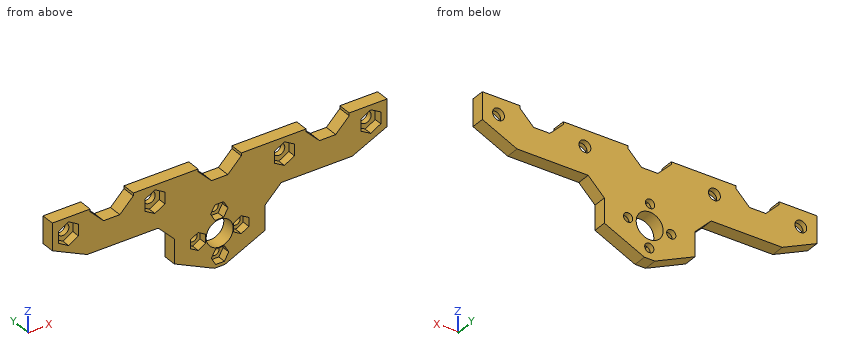
from build123d import *
from OCP.BRepFilletAPI import BRepFilletAPI_MakeChamfer

# Parameters (mm, degrees)
SKETCH1_W           = 124
SKETCH1_H           = 42
BOSS_EXTRUDE1_DEPTH = 5
SKETCH2_R           = 5
CUT_EXTRUDE1_DEPTH  = 5
SKETCH3_W           = 124
SKETCH3_H           = 42
SKETCH3_R           = 2.2
SKETCH3_R_2         = 1.7
SKETCH3_R_3         = 5
BOSS_EXTRUDE2_DEPTH = 2
CHAMFER1_SIZE       = 28
CHAMFER1_SIZE2      = 60.046193774
CUT_EXTRUDE2_DEPTH  = 10
LPATTERN1_COUNT     = 3
LPATTERN1_PITCH     = 40
SKETCH5_W           = 124
SKETCH5_H           = 4
CUT_EXTRUDE3_DEPTH  = 10
CUT_EXTRUDE4_DEPTH  = 10
CHAMFER2_SIZE       = 6


with BuildPart() as part:
    # Sketch1 → Boss-Extrude1 (new body)
    with BuildSketch(Plane.XZ.offset(-139.173467121)):
        with Locations((90.436218841, 110.61857787)):
            Rectangle(SKETCH1_W, SKETCH1_H)
        Polygon((87.341918286, 93.619783108), (88.95849904, 90.819783108), (92.191660547, 90.819783108), (93.808241301, 93.619783108), (92.191660547, 96.419783108), (88.95849904, 96.419783108), align=None, mode=Mode.SUBTRACT)
        Polygon((98.435013602, 98.524277315), (101.235013602, 100.140858069), (101.235013602, 103.374019576), (98.435013602, 104.99060033), (95.635013602, 103.374019576), (95.635013602, 100.140858069), align=None, mode=Mode.SUBTRACT)
        Polygon((82.437424079, 104.712878424), (79.637424079, 103.09629767), (79.637424079, 99.863136163), (82.437424079, 98.246555409), (85.237424079, 99.863136163), (85.237424079, 103.09629767), align=None, mode=Mode.SUBTRACT)
        Polygon((93.530519395, 109.617372631), (91.913938641, 112.417372631), (88.680777134, 112.417372631), (87.06419638, 109.617372631), (88.680777134, 106.817372631), (91.913938641, 106.817372631), align=None, mode=Mode.SUBTRACT)
        Polygon((34.436218841, 125.890969862), (30.736218841, 123.754773866), (30.736218841, 119.482381874), (34.436218841, 117.346185878), (38.136218841, 119.482381874), (38.136218841, 123.754773866), align=None, mode=Mode.SUBTRACT)
        Polygon((62.736218841, 123.754773866), (62.736218841, 119.482381874), (66.436218841, 117.346185878), (70.136218841, 119.482381874), (70.136218841, 123.754773866), (66.436218841, 125.890969862), align=None, mode=Mode.SUBTRACT)
        Polygon((118.136218841, 123.754773866), (114.436218841, 125.890969862), (110.736218841, 123.754773866), (110.736218841, 119.482381874), (114.436218841, 117.346185878), (118.136218841, 119.482381874), align=None, mode=Mode.SUBTRACT)
        Polygon((142.736218841, 119.482381874), (146.436218841, 117.346185878), (150.136218841, 119.482381874), (150.136218841, 123.754773866), (146.436218841, 125.890969862), (142.736218841, 123.754773866), align=None, mode=Mode.SUBTRACT)
    extrude(amount=BOSS_EXTRUDE1_DEPTH)

    # Sketch2 → Cut-Extrude1 (cut)
    with BuildSketch(Plane(origin=(0, 139.173467121, 0), x_dir=(1, 0, 0), z_dir=(0, 1, 0))):
        with Locations(Location((90.436218841, -101.61857787, 0), (0, 0, 270))):
            Circle(SKETCH2_R)
    extrude(amount=-CUT_EXTRUDE1_DEPTH, mode=Mode.SUBTRACT)

    # Sketch3 → Boss-Extrude2 (add)
    with BuildSketch(Plane(origin=(0, 139.173467121, 0), x_dir=(1, 0, 0), z_dir=(0, 1, 0))):
        with Locations((90.436218841, -110.61857787)):
            Rectangle(SKETCH3_W, SKETCH3_H)
        with Locations(Location((34.436218841, -121.61857787, 0), (0, 0, 270))):
            Circle(SKETCH3_R, mode=Mode.SUBTRACT)
        with Locations(Location((66.436218841, -121.61857787, 0), (0, 0, 270))):
            Circle(SKETCH3_R, mode=Mode.SUBTRACT)
        with Locations(Location((114.436218841, -121.61857787, 0), (0, 0, 270))):
            Circle(SKETCH3_R, mode=Mode.SUBTRACT)
        with Locations(Location((146.436218841, -121.61857787, 0), (0, 0, 270))):
            Circle(SKETCH3_R, mode=Mode.SUBTRACT)
        with Locations(Location((90.575079793, -93.619783108, 0), (0, 0, 270))):
            Circle(SKETCH3_R_2, mode=Mode.SUBTRACT)
        with Locations(Location((82.437424079, -101.479716917, 0), (0, 0, 270))):
            Circle(SKETCH3_R_2, mode=Mode.SUBTRACT)
        with Locations(Location((90.297357888, -109.617372631, 0), (0, 0, 270))):
            Circle(SKETCH3_R_2, mode=Mode.SUBTRACT)
        with Locations(Location((98.435013602, -101.757438823, 0), (0, 0, 270))):
            Circle(SKETCH3_R_2, mode=Mode.SUBTRACT)
        with Locations(Location((90.436218841, -101.61857787, 0), (0, 0, 270))):
            Circle(SKETCH3_R_3, mode=Mode.SUBTRACT)
    extrude(amount=-BOSS_EXTRUDE2_DEPTH)

    # Chamfer1: one chamfer whose edges measure the first distance from different faces: ONE call of the kernel's chamfer builder (chamfer() names one face for all edges)
    chamfer1_edges_1 = [part.edges().sort_by_distance(p)[0] for p in [
        (152.436218841, 136.673467121, 89.61857787),
    ]]
    chamfer1_side_1 = [part.faces().sort_by_distance(p)[0] for p in [
        (152.436218841, 136.673467121, 110.61857787),
    ]]
    chamfer1_edges_2 = [part.edges().sort_by_distance(p)[0] for p in [
        (28.436218841, 136.673467121, 89.61857787),
    ]]
    chamfer1_side_2 = [part.faces().sort_by_distance(p)[0] for p in [
        (28.436218841, 136.673467121, 110.61857787),
    ]]
    chamfer1 = BRepFilletAPI_MakeChamfer(part.part.solid().wrapped)
    for e in chamfer1_edges_1:
        chamfer1.Add(CHAMFER1_SIZE, CHAMFER1_SIZE2, e.wrapped, chamfer1_side_1[0].wrapped)  # the first distance lies on this face
    for e in chamfer1_edges_2:
        chamfer1.Add(CHAMFER1_SIZE, CHAMFER1_SIZE2, e.wrapped, chamfer1_side_2[0].wrapped)  # the first distance lies on this face
    add(Compound.cast(chamfer1.Shape()), mode=Mode.REPLACE)

    # Sketch4 → Cut-Extrude2 (cut)
    with BuildSketch(Plane.XZ.offset(-134.173467121)):
        Polygon((42.436218841, 131.61857787), (58.436218841, 131.61857787), (58.436218841, 126.61857787), (53.436218841, 121.61857787), (47.436218841, 121.61857787), (42.436218841, 126.61857787), align=None)
    cut_extrude2 = extrude(amount=-CUT_EXTRUDE2_DEPTH, mode=Mode.SUBTRACT)

    # LPattern1: Cut-Extrude2 ×3
    with Locations(*[(i * LPATTERN1_PITCH, 0, 0) for i in range(1, LPATTERN1_COUNT)]):
        add(cut_extrude2, mode=Mode.SUBTRACT)

    # Sketch5 → Cut-Extrude3 (cut)
    with BuildSketch(Plane.XZ.offset(-134.173467121)):
        with Locations((90.436218841, 129.61857787)):
            Rectangle(SKETCH5_W, SKETCH5_H)
    extrude(amount=-CUT_EXTRUDE3_DEPTH, mode=Mode.SUBTRACT)

    # Sketch6 → Cut-Extrude4 (cut)
    with BuildSketch(Plane.XZ.offset(-134.173467121)):
        Polygon((41.303260364, 111.61857787), (73.637424079, 111.61857787), (73.637424079, 96.540909709), align=None)
        Polygon((107.235013602, 111.61857787), (107.235013602, 96.540909709), (139.569177317, 111.61857787), align=None)
    extrude(amount=-CUT_EXTRUDE4_DEPTH, mode=Mode.SUBTRACT)

    # Chamfer2
    chamfer2_edges = [part.edges().sort_by_distance(p)[0] for p in [
        (73.637424079, 136.673467121, 111.61857787),
        (107.235013602, 136.673467121, 111.61857787),
    ]]
    chamfer(chamfer2_edges, length=CHAMFER2_SIZE)


solid = part.part
The listing builds one solid part. Answer for the finished solid, in the listing's coordinates (mm). Coordinates: 2 decimals unless noted, no trailing zeros. Order: outer loops, then holes, each group sorted by start corner. A loop starts at its lowest first (then second) coordinate and runs counter-clockwise, first axis right, second up.
Q1. A cutting plane is placed at B-B, the plane y = 138.3. State how many separate pieces and enclosed holes the cut face has, and give its area (3 significant figures).
Q2. Given P1, Ø2.5, axis at x = 130.5, y = 137, coming from the +Z side; P2, Ø1.5, axis at x = 132, y = 137.5, coming from the -Z side; P3, Ø1.7, axis at x = 99, z = 102.5, coming from the -Y side, each flat-ended and moving along its own axis, determine where each tip first touches the part or whether it passes through.
Q3. A cutting plane is placed at C-C, the plane x = 60. Write down the section's boundary in (y, z), and give its area (3 significant figures).
Q4. A cutting plane is placed at A-A, the plane z = 102. Write down the section's boundary in (x, y).
Q5. A cutting plane is placed at D-D, the plane z = 113.5. Write down the section's boundary in (x, y), and give its area (3 significant figures).
Q6. Consider line 1 (X direction, y = 138, z = 121.5); line 2 (X direction, y = 135.75, z = 121); line 3 (X direction, y = 136.95, z = 100.5). Determine where each line is inside the solid, lowest interval first.
Answers follow:
1. separate pieces: 1
1. enclosed holes: 9
1. area: 2,190 mm2
2. P1: stops at z = 121.62
2. P2: stops at z = 111.62
2. P3: stops at y = 137.17
3. outline: (134.17, 111.62) - (139.17, 111.62) - (139.17, 127.62) - (134.17, 127.62) - close
3. area: 80.0 mm2
4. outline: (73.64, 134.17) - (79.64, 134.17) - (79.64, 137.17) - (80.82, 137.17) - (80.82, 139.17) - (73.64, 139.17) - close; (84.06, 137.17) - (85.24, 137.17) - (85.24, 134.17) - (85.45, 134.17) - (85.45, 139.17) - (84.06, 139.17) - close; (95.42, 134.17) - (95.64, 134.17) - (95.64, 137.17) - (96.75, 137.17) - (96.75, 139.17) - (95.42, 139.17) - close; (100.12, 137.17) - (101.24, 137.17) - (101.24, 134.17) - (107.24, 134.17) - (107.24, 139.17) - (100.12, 139.17) - close
5. outline: (37.27, 134.17) - (143.6, 134.17) - (143.6, 139.17) - (37.27, 139.17) - close
5. area: 532 mm2
6. line 1: x = 28.44 to 32.24, 36.63 to 64.24, 68.63 to 112.24, 116.63 to 144.24, 148.63 to 152.44
6. line 2: x = 28.44 to 30.74, 38.14 to 62.74, 70.14 to 110.74, 118.14 to 142.74, 150.14 to 152.44
6. line 3: x = 73.64 to 79.64, 85.24 to 85.56, 95.31 to 95.64, 101.24 to 107.24
